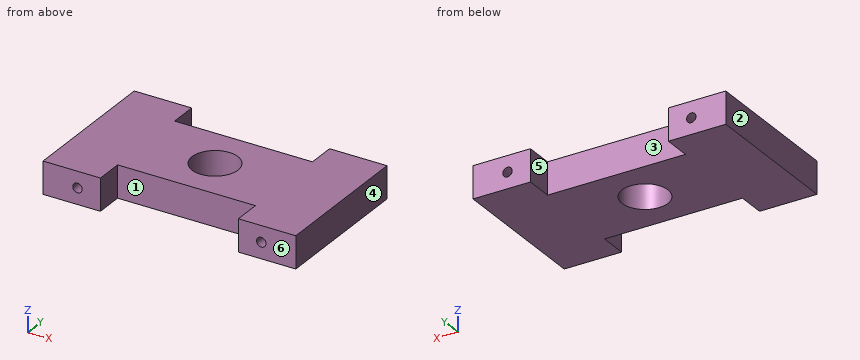
```python
from build123d import *

# Parameters (mm, degrees)
SKETCH1_R                = 5
BOSS_EXTRUDE1_DEPTH      = 7
M2_5X0_45_TAPPED_HOLE1_D = 2.05


with BuildPart() as part:
    # Sketch1 → Boss-Extrude1 (new body)
    with BuildSketch(Plane.XY):
        Polygon((-15, 10), (-15, 16), (-27.5, 16), (-27.5, -16), (-15, -16), (-15, -10), (15, -10), (15, -16), (27.5, -16), (27.5, 16), (15, 16), (15, 10), align=None)
        Circle(SKETCH1_R, mode=Mode.SUBTRACT)
    extrude(amount=BOSS_EXTRUDE1_DEPTH)

    # M2.5x0.45 Tapped Hole1 (through all)
    with Locations(Plane(origin=(0, 16, 0), x_dir=(-1, 0, 0), z_dir=(0, 1, 0))):
        with Locations((20, 3.5), (-20, 3.5)):
            Hole(M2_5X0_45_TAPPED_HOLE1_D / 2)


solid = part.part
```
Input: part model. Units: mm. Frame: model coordinates. Face numbers are marked on the shaded views. A direction names the side the tool comes from. Coordinates: 2 decimals unless noted, no trailing zeros. Loops run counter-clockwise (first coordinate to the right, second up) from the corner with the lowest first, then second, coordinate; pieces in that order, holes last.
Q1. Line query: line 1 along X through (y, z) = (-14, 6.25); line 2 along Y through (x, z) = (0, 4); line 3 along Y through (x, z) = (14, 3.5). Output: solid intervals per line, ascending.
Results are:
line 1: x = -27.5 to -15, 15 to 27.5
line 2: y = -10 to -5, 5 to 10
line 3: y = -10 to 10
Q2. Contact query for a flat-ended pin moving along its axis: pin 1 (8 mm diameter, centred on x = 0, y = 0, fed in from -Z). Output: stop coordinate, or through.
Results are:
pin 1: passes through
Q3. Section C-C, the plane y = 4. Return the cut outline in (x, z) (3 decimals), and give its area (3 significant figures).
Results are:
outline: (-27.5, 0) - (-3, 0) - (-3, 7) - (-27.5, 7) - close; (3, 0) - (27.5, 0) - (27.5, 7) - (3, 7) - close; hole circle Ø2.05 at (-20, 3.5); hole circle Ø2.05 at (20, 3.5)
area: 336 mm2
Q4. Mould query, pull axis X, two halves, no side actions, for the marked faces 4, 5 and 6. Classes: +X half, -X half, draft (parallel to the pull), parting line (faces both ways), or undercut.
Results are:
face 4: +X half
face 5: undercut
face 6: draft
Q5. Section B-B, the plane z = 3.5. Return the cut outline in (x, y) (3 decimals).
Results are:
outline: (-27.5, -16) - (-21.025, -16) - (-21.025, 16) - (-27.5, 16) - close; (-18.975, -16) - (-15, -16) - (-15, -10) - (15, -10) - (15, -16) - (18.975, -16) - (18.975, 16) - (15, 16) - (15, 10) - (-15, 10) - (-15, 16) - (-18.975, 16) - close; (21.025, -16) - (27.5, -16) - (27.5, 16) - (21.025, 16) - close; hole circle Ø10 at (0, 0)
Q6. Section A-A, the plane x = -20. Return the cut outline in (y, z) (3 decimals), and give its area (3 significant figures).
Results are:
outline: (-16, 0) - (16, 0) - (16, 2.475) - (-16, 2.475) - close; (-16, 4.525) - (16, 4.525) - (16, 7) - (-16, 7) - close
area: 158 mm2
Q7. Set-up query: the marked faces 1, 2 and 3. Return all of +Z, -Z, +X, -X, +Y, -Y with unobstructed straight access to the full face (end or side cutting, diameter ignored); none if empty.
Results are:
face 1: +Z, -Z, -Y
face 2: +Z, -Z, -X, +Y, -Y
face 3: +Z, -Z, +Y
Q8. Section D-D, the plane y = -2.5. Return the cut outline in (x, z) (3 decimals), and give its area (3 significant figures).
Results are:
outline: (-27.5, 0) - (-4.33, 0) - (-4.33, 7) - (-27.5, 7) - close; (4.33, 0) - (27.5, 0) - (27.5, 7) - (4.33, 7) - close; hole circle Ø2.05 at (-20, 3.5); hole circle Ø2.05 at (20, 3.5)
area: 318 mm2
